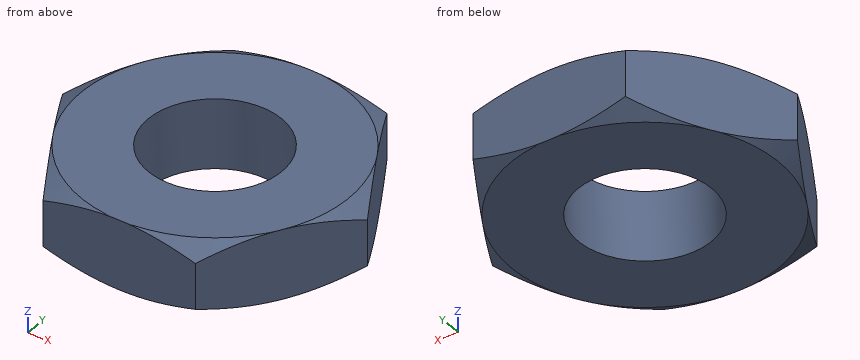
Solid Edge part; units mm, degrees
sketch "Sketch1" plane through (0, 0, 0) normal (0, 0, 1) x (1, 0, 0)
  line L0 (-10, -17.3205) -> (10, -17.3205)
  line L1 (10, -17.3205) -> (20, 0)
  line L2 (20, 0) -> (10, 17.3205)
  line L3 (10, 17.3205) -> (-10, 17.3205)
  line L4 (-10, 17.3205) -> (-20, 0)
  line L5 (-20, 0) -> (-10, -17.3205)
  dimension "D1" = 10
extrude "Protrusion1" add sketch "Sketch1" along normal mid plane 9
hole "Hole_1" at (0, 0, 4.5) direction (0, 0, -1) diameter 17.294 end through all
sketch "Sketch2" plane through (0, 0, 0) normal (1, 0, 0) x (0, 1, 0)
  line L0 (17.3205, -4.5) -> (44.5217, 11.2046)
revolve "RevolvedCutout1" cut sketch "Sketch2" angle 360 about axis through (0, 0, -57) along (0, 0, 1) material side at (0, 30.9461, 3.309)
mirror "Mirror1" about plane through (0, 0, 0) normal (0, 0, 1) of "RevolvedCutout1"
properties part number "5" material "Fe 410 W"
Input: part model. Units: mm. Frame: model coordinates. Coordinates: 2 decimals unless noted, no trailing zeros. Write each loop counter-clockwise with the first axis right and the second up, starting at its lowest first coordinate (ties: lowest second). Pieces come first, ordered by that corner, then holes. Notation, with made-up numbers: (52, 56) - (57, 56) arc R32 cw to (57, 94) - close; hole circle Ø1 at (23.5, -38.5). An arc over 180 degrees is marked (long way). Put each result on its own line as item: value. Start each with the question number.
1) Cut plane A-A (z = 0.75). Return the cut outline in (x, y), plus the area to 3 significant figures.
2) Cut plane B-B (z = -3.5). Return the cut outline in (x, y), plus the area to 3 significant figures.
3) Contact query for flat-ended pins moving along their axis: pin 1 (20 mm diameter, centred on x = 0, y = 0, fed in from +Z); pin 2 (1 mm diameter, centred on x = -12.5, y = -13.5, fed in from -Z). Output: stop coordinate, or through.
4) Ray query, L1, parallel to Y at x = 0, z = 2; L2, parallel to X at y = 0, z = 1.5; L3, parallel to X at y = 5.5, z = 1. Return the intervals inside material, ascending.
Resolved:
1. outline: (-20, 0) - (-10, -17.32) - (10, -17.32) - (20, 0) - (10, 17.32) - (-10, 17.32) - close; hole circle Ø17.29 at (0, 0)
1. area: 804 mm2
2. outline: (-18.97, -1.79) - (-11.03, -15.53) arc R19.05 ccw to (-7.94, -17.32) - (7.94, -17.32) arc R19.05 ccw to (11.03, -15.53) - (18.97, -1.79) arc R19.05 ccw to (18.97, 1.79) - (11.03, 15.53) arc R19.05 ccw to (7.94, 17.32) - (-7.94, 17.32) arc R19.05 ccw to (-11.03, 15.53) - (-18.97, 1.79) arc R19.05 ccw to start; hole circle Ø17.29 at (0, 0)
2. area: 794 mm2
3. pin 1: stops at z = 4.5
3. pin 2: stops at z = -4.17
4. L1: y = -17.32 to -8.65, 8.65 to 17.32
4. L2: x = -20 to -8.65, 8.65 to 20
4. L3: x = -16.82 to -6.67, 6.67 to 16.82
